Can you work these out from the drawing? Everything is in mm from the part's minimum corner. Round coordinates to 2 decimals unless told otherwise and drop trailing zeros. Order: outer loops, then holes, each group sorted by start corner. A loop starts at its lowest first (then second) coordinate and runs counter-clockwise, first axis right, second up. Notation, with made-up numbers: (24, -25) -> (67, -25) arc R28 ccw to (67, 2) -> close; hole circle Ø5 at (32, 55). An arc over 180 degrees is marked (long way). One line per item, written item: value.
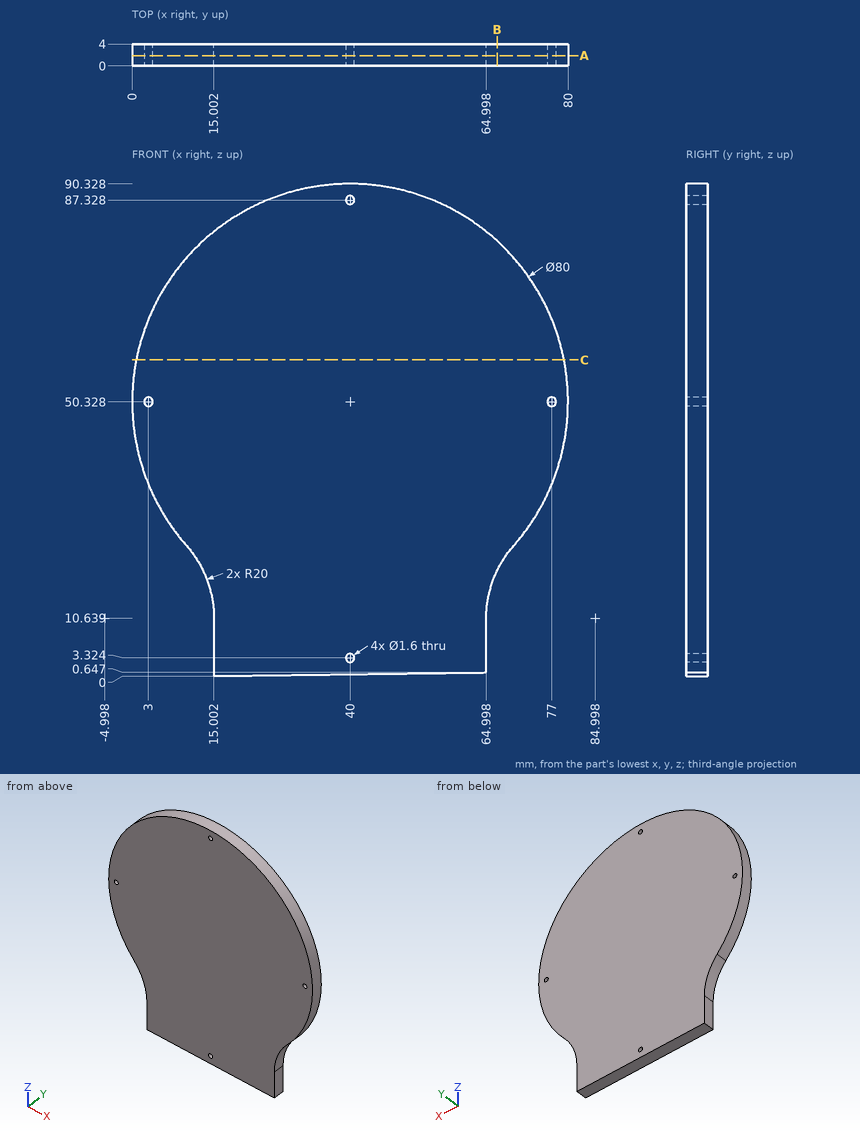
Q1. I want a section at A-A on y = 1.85. Write out the boundary of the cut face in (x, z).
Answers:
outline: (10, 23.87) arc R20 cw to (15, 10.64) -> (15, 0) -> (65, 0.65) -> (65, 10.64) arc R20 cw to (70, 23.87) arc R40 ccw (long way) to start; hole circle Ø1.6 at (3, 50.33); hole circle Ø1.6 at (40, 3.32); hole circle Ø1.6 at (40, 87.33); hole circle Ø1.6 at (77, 50.33)
Q2. I want a section at C-C on z = 58. Write out the boundary of the cut face in (x, y).
Answers:
outline: (0.74, 0) -> (79.26, 0) -> (79.26, 4) -> (0.74, 4) -> close
Q3. I need wall thicknesses on line 1 along Z through (x, y) = (40, 2.9); line 2 along X through (y, z) = (0.4, 10.5); line 3 along X through (y, z) = (0.85, 16.5) (1 decimal). Which ranges of each line are inside material? Lowest first, please.
Answers:
line 1: 0.32 to 2.52, 4.12 to 86.53, 88.13 to 90.33
line 2: 15 to 65
line 3: 14.1 to 65.9
Q4. I want a section at B-B on x = 67. Write out the boundary of the cut face in (y, z).
Answers:
outline: (0, 19.36) -> (4, 19.36) -> (4, 79.84) -> (0, 79.84) -> close
Q5. For P1, Ø1, axis at y = 3.5, z = 9, coming from the +X side; P2, Ø2, axis at y = 1, z = 8, coming from the -X side; P3, Ø1.5, axis at y = 2.5, z = 46.5, coming from the +X side, each with a flat end and sliding along its axis, tell me the tip position at first contact or that it passes through.
Answers:
P1: x = 65
P2: x = 15
P3: x = 79.88
